from build123d import *
from build123d.topology import SkipClean

# Parameters (mm, degrees)
ESQUISSE2_R             = 10
EXTRUSION1_DEPTH        = 15
ENL_V_START             = -1
ENL_V_MAT_EXTRU_1_DEPTH = 1
EXTRUSION2_DEPTH        = 1
ESQUISSE5_W             = 3
ESQUISSE5_H             = 20


with BuildPart() as part:
    # Esquisse1 → Révolution1 (revolve)
    with BuildSketch(Plane.XY):
        Polygon((-54, 15), (-54, 0), (73, 0), (73, 12), (-32, 12), (-32, 8.364637375), (-52, 8.364637375), (-52, 15), align=None)
    revolve(axis=Axis((-54, 0, 0), (1, 0, 0)))

    # Esquisse2 → Extrusion1 (add)
    with BuildSketch(Plane(origin=(73, 0, 0), x_dir=(0, 0, -1), z_dir=(1, 0, 0))):
        with Locations(Location((0, 0, 0), (0, 0, 90))):
            Circle(ESQUISSE2_R)
    extrude(amount=EXTRUSION1_DEPTH)

    # Esquisse3 → Enlèv. mat.-Extru.1 (cut)
    with BuildSketch(Plane(origin=(88, 0, 0), x_dir=(0, 0, -1), z_dir=(1, 0, 0)).offset(ENL_V_START)):
        with BuildLine():
            Line((2, -9.797958971), (2, 9.797958971))
            ThreePointArc((2, 9.797958971), (-10, 0), (2, -9.797958971))
        make_face()
    extrude(amount=ENL_V_MAT_EXTRU_1_DEPTH, mode=Mode.SUBTRACT)

    # Esquisse4 → Extrusion2 (add)
    with SkipClean():  # the faces are left unmerged after this step: merging them gives an invalid solid
        with BuildSketch(Plane(origin=(87, 0, 0), x_dir=(0, 0, -1), z_dir=(1, 0, 0))):
            with BuildLine():
                Line((-2, 9.797958971), (-2, -9.797958971))
                ThreePointArc((-2, -9.797958971), (-10, 0), (-2, 9.797958971))
            make_face()
        extrude(amount=EXTRUSION2_DEPTH)

    # Esquisse5 → Enlèvement de matière-Révolution1 (revolve, cut)
    with BuildSketch(Plane.XY, mode=Mode.PRIVATE) as enl_vement_de_mati_re_r_volution1_sk:
        with Locations((81, 0)):
            Rectangle(ESQUISSE5_W, ESQUISSE5_H)
    revolve(enl_vement_de_mati_re_r_volution1_sk.sketch.rotate(Axis((82.5, -10, 0), (0, 1, 0)), 90), axis=Axis((82.5, -10, 0), (0, 1, 0)), mode=Mode.SUBTRACT)


solid = part.part
Verification items for the finished model (mm, model axes). A direction names the side the tool comes from. Round coordinates to 2 decimals unless told otherwise and drop trailing zeros. Order: outer loops, then holes, each group sorted by start corner. A loop starts at its lowest first (then second) coordinate and runs counter-clockwise, first axis right, second up.
1. Section check D-D on x = 82.5. Record the cut outline in (y, z), then the cut area to 3 significant figures.
Final values:
outline: (-9.54, -3) arc R10 ccw to (9.54, -3) - close; (-9.54, 3) - (9.54, 3) arc R10 ccw to start
area: 196 mm2
2. Section check B-B on y = 0. Record the cut outline in (x, z), then the cut area to 3 significant figures.
Final values:
outline: (-54, -15) - (-52, -15) - (-52, -8.36) - (-32, -8.36) - (-32, -12) - (73, -12) - (73, -10) - (88, -10) - (88, -2) - (87, -2) - (87, 2) - (88, 2) - (88, 10) - (73, 10) - (73, 12) - (-32, 12) - (-32, 8.36) - (-52, 8.36) - (-52, 15) - (-54, 15) - close; hole circle Ø6 at (82.5, 0)
area: 3,180 mm2
3. Section check C-C on z = 5.5. Record the cut outline in (x, y), then the cut area to 3 significant figures.
Final values:
outline: (-54, -13.96) - (-52, -13.96) - (-52, -6.3) - (-32, -6.3) - (-32, -10.67) - (73, -10.67) - (73, -8.35) - (88, -8.35) - (88, 8.35) - (73, 8.35) - (73, 10.67) - (-32, 10.67) - (-32, 6.3) - (-52, 6.3) - (-52, 13.96) - (-54, 13.96) - close
area: 2,800 mm2
4. Access from +Z, -Z, +X, -X, +Y, -Y to the whole of each face (thin tool, end or side, straight path). Record for faces 1 (the flat face through (88, 0, -5)), 2 (the flat face through (-54, 0, 0)), 3 (the flat face through (87, 0, 0)), 4 (the flat face through (-52, -6.5, -6.5)), 5 (the flat face through (73, 5, 9)).
Final values:
face 1: +Z, -Z, +X, +Y, -Y
face 2: +Z, -Z, -X, +Y, -Y
face 3: +X, +Y, -Y
face 4: none
face 5: +X
5. Go/stop test with flat-tipped pins: P1, Ø8, axis at x = 51, z = 7.5, coming from the -Y side; P2, Ø1.5, axis at x = -12, z = 5, coming from the -Y side; P3, Ø7, axis at x = 82.5, z = 0, coming from the -Y side. Record where each tip stops, or that it passes through.
Final values:
P1: stops at y = -11.48
P2: stops at y = -11.22
P3: stops at y = -10
6. Thickness scan on L1, parallel to X at y = 1.5, z = 0; L2, parallel to X at y = 3.5, z = 8.5; L3, parallel to X at y = 8.5, z = -1.75. Record the ranges inside material, lowest first.
Final values:
L1: x = -54 to 79.5, 85.5 to 87
L2: x = -54 to -52, -32 to 88
L3: x = -54 to -52, -32 to 80.06, 84.94 to 87
7. Release check for a two-part mould opening along X. For faces 6 (the flat face through (88, 0, 5)), 7 (the cylindrical face through (-53.014, -14.985, 0.66)), 8 (the cylindrical face through (79.57, 0.14, -0.65)) record: +X half, -X half, draft (parallel to the pull), parting line (faces both ways), or undercut.
Final values:
face 6: +X half
face 7: draft
face 8: undercut
8. Section check A-A on z = 0. Record the cut outline in (x, y), then the cut area to 3 significant figures.
Final values:
outline: (-54, -15) - (-52, -15) - (-52, -8.36) - (-32, -8.36) - (-32, -12) - (73, -12) - (73, -10) - (79.5, -10) - (79.5, 10) - (73, 10) - (73, 12) - (-32, 12) - (-32, 8.36) - (-52, 8.36) - (-52, 15) - (-54, 15) - close; (85.5, -10) - (87, -10) - (87, 10) - (85.5, 10) - close
area: 3,070 mm2
